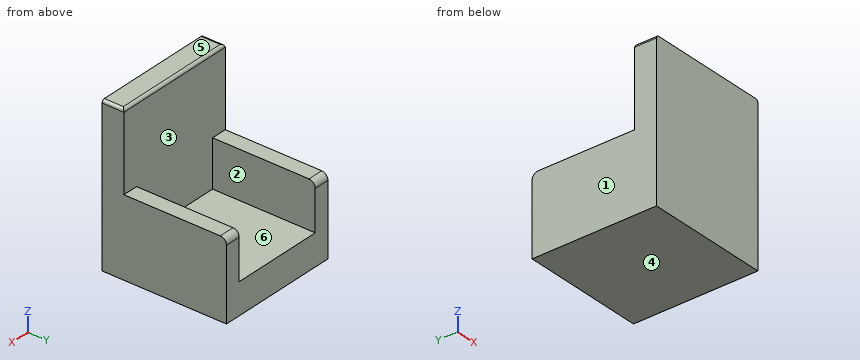
from build123d import *

# Parameters (mm, degrees)
F0_W     = 101.6
F0_H     = 101.6
F1_DEPTH = 25.4
F2_W     = 101.6
F2_H     = 17.786168
F3_DEPTH = 101.6
F4_W     = 12.7
F4_H     = 83.813832
F5_DEPTH = 38.1
F6_R     = 5.08
F7_R     = 5.08
F8_R     = 2.286


with BuildPart() as f1:
    # F0 (on Top) → F1 (new body)
    with BuildSketch(Plane.XY):
        with Locations((0.158782, 3.229056)):
            Rectangle(F0_W, F0_H)
    extrude(amount=F1_DEPTH)

    # F2 (on face) → F3 (join)
    with BuildSketch(Plane.XY.offset(25.4)):
        with Locations((0.158782, -38.67786)):
            Rectangle(F2_W, F2_H)
    extrude(amount=F3_DEPTH)

    # F4 (on face) → F5 (join)
    with BuildSketch(Plane.XY.offset(25.4)):
        with Locations((44.608782, 12.12214)):
            Rectangle(F4_W, F4_H)
        with Locations((-44.291218, 12.12214)):
            Rectangle(F4_W, F4_H)
    extrude(amount=F5_DEPTH)

    # F6
    f6_edges = [f1.edges().sort_by_distance(p)[0] for p in [
        (44.608782, 54.029056, 63.5),
    ]]
    fillet(f6_edges, radius=F6_R)

    # F7
    f7_edges = [f1.edges().sort_by_distance(p)[0] for p in [
        (-44.291218, 54.029056, 63.5),
    ]]
    fillet(f7_edges, radius=F7_R)

    # F8
    f8_edges = [f1.edges().sort_by_distance(p)[0] for p in [
        (0.158782, -29.784776, 127),
        (-50.641218, -38.67786, 127),
        (50.958782, -38.67786, 127),
    ]]
    fillet(f8_edges, radius=F8_R)


solid = f1.part
Model file for the job. Use its own axes, mm. Face numbers are marked on the shaded views. A direction names the side the tool comes from. Give positions to 0.01 mm unless a question says otherwise; leave off trailing zeros. Order: outer loops, then holes, each group sorted by start corner. A loop starts at its lowest first (then second) coordinate and runs counter-clockwise, first axis right, second up. Notation, with made-up numbers: (13, -28) - (51, -28) arc R11 cw to (51, -15) - close; hole circle Ø10 at (32.25, -25). An arc over 180 degrees is marked (long way). One line per item, written item: value.
Item 1: Pin check, flat tips, straight feed: pin 1 Ø3 at (x, y) = (-9.5, -17) entering from +Z; pin 2 Ø12 at (x, z) = (1, 104) entering from +Y; pin 3 Ø14 at (x, y) = (45, -2) entering from +Z. Stop position of each tip, or through.
Response values:
pin 1: z = 25.4
pin 2: y = -29.78
pin 3: z = 63.5
Item 2: Slice it at C-C (x = 23). List the corners of the cut face in (y, z), then the cut area to 3 significant figures.
Response values:
outline: (-47.57, 0) - (54.03, 0) - (54.03, 25.4) - (-29.78, 25.4) - (-29.78, 124.71) arc R2.29 ccw to (-32.07, 127) - (-47.57, 127) - close
area: 4,390 mm2
Item 3: Two-plate mould, pull along X, no slides. Class the marked faces 1, 2, 3 and 4: released by +X, released by -X, zero draft, split by the parting line, or undercut.
Response values:
face 1: released by -X
face 2: undercut
face 3: undercut
face 4: zero draft
Item 4: Slice it at D-D (z = 115.5). List the corners of the cut face in (x, y), then the cut area to 3 significant figures.
Response values:
outline: (-50.64, -47.57) - (50.96, -47.57) - (50.96, -29.78) - (-50.64, -29.78) - close
area: 1,810 mm2
Item 5: Slice it at A-A (z = 47.5). List the corners of the cut face in (x, y), then the cut area to 3 significant figures.
Response values:
outline: (-50.64, -47.57) - (50.96, -47.57) - (50.96, 54.03) - (38.26, 54.03) - (38.26, -29.78) - (-37.94, -29.78) - (-37.94, 54.03) - (-50.64, 54.03) - close
area: 3,940 mm2
Item 6: Tool access for the marked faces 5 and 6: list every direction of +Z, -Z, +X, -X, +Y, -Y with a clear straight run to the whole face (end or side of a thin tool).
Response values:
face 5: +Z, +X, -X, +Y, -Y
face 6: +Z, +Y
Item 7: Wall check: line 1 (X direction, y = 32, z = 39); line 2 (Z direction, x = -31, y = 32.5); line 3 (Y direction, x = -6, z = 40). Give the ranges that are in metal, low to high.
Response values:
line 1: -50.64 to -37.94, 38.26 to 50.96
line 2: 0 to 25.4
line 3: -47.57 to -29.78
Item 8: Slice it at B-B (x = 44). List the corners of the cut face in (y, z), then the cut area to 3 significant figures.
Response values:
outline: (-47.57, 0) - (54.03, 0) - (54.03, 58.42) arc R5.08 ccw to (48.95, 63.5) - (-29.78, 63.5) - (-29.78, 124.71) arc R2.29 ccw to (-32.07, 127) - (-47.57, 127) - close
area: 7,570 mm2
